```python
from build123d import *

# Parameters (mm, degrees)
EXTRUDE_1_DEPTH             = 25
EXTRUDE_3_DEPTH             = 25
CUT_EXTRUDE_1_DEPTH         = 53.179559149
CUT_EXTRUDE_1_DEPTH_BACK    = 53.179559149
SKETCH_4_W                  = 32
SKETCH_4_H                  = 14.912747354
FILLET_1_R                  = 10
FILLET_17_R                 = 2
CUT_EXTRUDE_5_DEPTH         = 60.625850278
CUT_EXTRUDE_5_DEPTH_BACK    = 60.625850278
CUT_EXTRUDE_6_DEPTH         = 60.600832153
CUT_EXTRUDE_6_DEPTH_BACK    = 60.600832153
SKETCH_9_W                  = 7
SKETCH_9_H                  = 3
SKETCH_10_W                 = 4.226496159
SKETCH_10_H                 = 9
EXTRUDE_4_DEPTH             = 10
SKETCH_12_W                 = 50
SKETCH_12_H                 = 3
EXTRUDE_6_DEPTH             = 10
EXTRUDE_6_DIRECTION_2_REACH = 62.659
SKETCH_14_R                 = 1
CUT_EXTRUDE_8_DEPTH         = 64.621818473
FILLET_50_R                 = 1.32
SKETCH_16_W                 = 32
SKETCH_16_H                 = 21.912747354
EXTRUDE_7_DEPTH             = 4.226496158
EXTRUDE_START               = 32
EXTRUDE_8_DEPTH             = 32
CHAMFER_1_SIZE              = 3


with BuildPart() as part:
    # 草图1 → 凸台-拉伸1 (new, symmetric)
    with BuildSketch(Plane.XY):
        with BuildLine():
            ThreePointArc((-33, 0), (-29.908156972, 13.946402637), (-21.21199112, 25.279466623))
            Line((-21.21199112, 25.279466623), (-16.985494961, 24.909696123))
            Line((-16.985494961, 24.909696123), (-19.283628291, 22.981333294))
            ThreePointArc((-19.283628291, 22.981333294), (-27.189233611, 12.678547852), (-30, 0))
            Line((-30, 0), (-33, 0))
        make_face()
    extrude(amount=EXTRUDE_1_DEPTH, both=True)

    # 草图1<7> → 凸台-拉伸3 (add, symmetric)
    with BuildSketch(Plane.XY):
        Polygon((-21.21199112, 25.279466623), (-21.21199112, 39.909696123), (-28.21199112, 39.909696123), (-28.21199112, 42.909696123), (-16.985494961, 42.909696123), (-16.985494961, 39.909696123), (-16.985494961, 24.909696123), align=None)
    extrude(amount=EXTRUDE_3_DEPTH, both=True)

    # 草图4 → 切除-拉伸1 (cut, two sides: drawn at the far end of the back side and taken through both)
    with BuildSketch(Plane(origin=(-16.985494961, 0, 0), x_dir=(0, 0, -1), z_dir=(1, 0, 0)).offset(-CUT_EXTRUDE_1_DEPTH_BACK)):
        with Locations((0, 35.453322446)):
            Rectangle(SKETCH_4_W, SKETCH_4_H)
    extrude(amount=CUT_EXTRUDE_1_DEPTH + CUT_EXTRUDE_1_DEPTH_BACK, mode=Mode.SUBTRACT)

    # 圆角1
    # the kernel refuses this fillet: 10 mm, written as the material it adds along each edge
    with BuildSketch(Plane(origin=(-21.21199112, 25.279466623, 25), x_dir=(-0.7281290100330119, -0.6854401102564294, 0), z_dir=(0, 0, -1))) as fillet_1_piece_1_section:
        with BuildLine():
            CenterArc((4.335441405, 9.983715921), FILLET_1_R, 223.270229162, 43.459541677)
            Line((-2.945848695, 3.129314818), (0, 0))
            ThreePointArc((0, 0), (1.882494294, 0.053737462), (3.764988589, 0))
        make_face()
    fillet_1_piece_1 = extrude(amount=50, mode=Mode.PRIVATE)
    fillet_1_piece_1 = split(fillet_1_piece_1, bisect_by=Plane(origin=(-21.85438977, 25.398045646, 16), z_dir=(0, 0, 1)), keep=Keep.TOP, mode=Mode.PRIVATE)
    fillet_1_piece_1 = split(fillet_1_piece_1, bisect_by=Plane(origin=(-21.85438977, 27.996948769, 20.5), z_dir=(0, -1, 0)), keep=Keep.TOP, mode=Mode.PRIVATE)
    add(fillet_1_piece_1)
    with BuildSketch(Plane(origin=(-21.21199112, 25.279466623, 25), x_dir=(-0.7281290100330119, -0.6854401102564294, 0), z_dir=(0, 0, -1))) as fillet_1_piece_2_section:
        with BuildLine():
            CenterArc((4.335441405, 9.983715921), FILLET_1_R, 223.270229162, 43.459541677)
            Line((-2.945848695, 3.129314818), (0, 0))
            ThreePointArc((0, 0), (1.882494294, 0.053737462), (3.764988589, 0))
        make_face()
    fillet_1_piece_2 = extrude(amount=50, mode=Mode.PRIVATE)
    fillet_1_piece_2 = split(fillet_1_piece_2, bisect_by=Plane(origin=(-21.135777092, 28.718730095, 16), z_dir=(0, 0, 1)), keep=Keep.TOP, mode=Mode.PRIVATE)
    fillet_1_piece_2 = split(fillet_1_piece_2, bisect_by=Plane(origin=(-21.135777092, 27.996948769, 20.5), z_dir=(0, 1, 0)), keep=Keep.TOP, mode=Mode.PRIVATE)
    add(fillet_1_piece_2)
    with BuildSketch(Plane(origin=(-21.21199112, 25.279466623, 25), x_dir=(-0.7281290100330119, -0.6854401102564294, 0), z_dir=(0, 0, -1))) as fillet_1_piece_3_section:
        with BuildLine():
            CenterArc((4.335441405, 9.983715921), FILLET_1_R, 223.270229162, 43.459541677)
            Line((-2.945848695, 3.129314818), (0, 0))
            ThreePointArc((0, 0), (1.882494294, 0.053737462), (3.764988589, 0))
        make_face()
    fillet_1_piece_3 = extrude(amount=50, mode=Mode.PRIVATE)
    fillet_1_piece_3 = split(fillet_1_piece_3, bisect_by=Plane(origin=(-21.85438977, 25.398045646, 16), z_dir=(0, 0, -1)), keep=Keep.TOP, mode=Mode.PRIVATE)
    fillet_1_piece_3 = split(fillet_1_piece_3, bisect_by=Plane(origin=(-21.85438977, 27.996948769, 0), z_dir=(0, -1, 0)), keep=Keep.TOP, mode=Mode.PRIVATE)
    fillet_1_piece_3 = split(fillet_1_piece_3, bisect_by=Plane(origin=(-21.85438977, 25.398045646, -16), z_dir=(0, 0, 1)), keep=Keep.TOP, mode=Mode.PRIVATE)
    add(fillet_1_piece_3)
    with BuildSketch(Plane(origin=(-21.21199112, 25.279466623, 25), x_dir=(-0.7281290100330119, -0.6854401102564294, 0), z_dir=(0, 0, -1))) as fillet_1_piece_4_section:
        with BuildLine():
            CenterArc((4.335441405, 9.983715921), FILLET_1_R, 223.270229162, 43.459541677)
            Line((-2.945848695, 3.129314818), (0, 0))
            ThreePointArc((0, 0), (1.882494294, 0.053737462), (3.764988589, 0))
        make_face()
    fillet_1_piece_4 = extrude(amount=50, mode=Mode.PRIVATE)
    fillet_1_piece_4 = split(fillet_1_piece_4, bisect_by=Plane(origin=(-21.85438977, 27.996948769, -20.5), z_dir=(0, -1, 0)), keep=Keep.TOP, mode=Mode.PRIVATE)
    fillet_1_piece_4 = split(fillet_1_piece_4, bisect_by=Plane(origin=(-21.85438977, 25.398045646, -16), z_dir=(0, 0, -1)), keep=Keep.TOP, mode=Mode.PRIVATE)
    add(fillet_1_piece_4)
    with BuildSketch(Plane(origin=(-21.21199112, 25.279466623, 25), x_dir=(-0.7281290100330119, -0.6854401102564294, 0), z_dir=(0, 0, -1))) as fillet_1_piece_5_section:
        with BuildLine():
            CenterArc((4.335441405, 9.983715921), FILLET_1_R, 223.270229162, 43.459541677)
            Line((-2.945848695, 3.129314818), (0, 0))
            ThreePointArc((0, 0), (1.882494294, 0.053737462), (3.764988589, 0))
        make_face()
    fillet_1_piece_5 = extrude(amount=50, mode=Mode.PRIVATE)
    fillet_1_piece_5 = split(fillet_1_piece_5, bisect_by=Plane(origin=(-21.135777092, 27.996948769, -20.5), z_dir=(0, 1, 0)), keep=Keep.TOP, mode=Mode.PRIVATE)
    fillet_1_piece_5 = split(fillet_1_piece_5, bisect_by=Plane(origin=(-21.135777092, 28.718730095, -16), z_dir=(0, 0, -1)), keep=Keep.TOP, mode=Mode.PRIVATE)
    add(fillet_1_piece_5)

    # 圆角17
    fillet_17_edges = [part.edges().sort_by_distance(p)[0] for p in [
        (-16.985494961, 24.909696123, 0),
    ]]
    fillet(fillet_17_edges, radius=FILLET_17_R)

    # 草图7 → 切除-拉伸5 (cut, two sides: drawn at the far end of the back side and taken through both)
    with BuildSketch(Plane.XY.offset(-CUT_EXTRUDE_5_DEPTH_BACK)):
        with BuildLine():
            Line((0, 0), (-33, 0))
            ThreePointArc((-33, 0), (-32.988691724, 0.863839294), (-32.954774647, 1.727086556))
            Line((-32.954774647, 1.727086556), (0, 0))
        make_face()
    extrude(amount=CUT_EXTRUDE_5_DEPTH + CUT_EXTRUDE_5_DEPTH_BACK, mode=Mode.SUBTRACT)

    # 草图9 → 切除-拉伸6 (cut, two sides: drawn at the far end of the back side and taken through both)
    with BuildSketch(Plane.XY.offset(-CUT_EXTRUDE_6_DEPTH_BACK)):
        with Locations((-24.71199112, 41.409696123)):
            Rectangle(SKETCH_9_W, SKETCH_9_H)
    extrude(amount=CUT_EXTRUDE_6_DEPTH + CUT_EXTRUDE_6_DEPTH_BACK, mode=Mode.SUBTRACT)

    # 草图10 → 凸台-拉伸4 (add)
    with BuildSketch(Plane(origin=(0, 42.909696123, 0), x_dir=(1, 0, 0), z_dir=(0, 1, 0))):
        with Locations((-19.098743041, 20.5)):
            Rectangle(SKETCH_10_W, SKETCH_10_H)
        with Locations((-19.098743041, -20.5)):
            Rectangle(SKETCH_10_W, SKETCH_10_H)
    extrude(amount=EXTRUDE_4_DEPTH)

    # 草图12 → 凸台-拉伸6 (add)
    with BuildSketch(Plane(origin=(-16.985494961, 0, 0), x_dir=(0, 0, -1), z_dir=(1, 0, 0))):
        with Locations((0, 51.409696123)):
            Rectangle(SKETCH_12_W, SKETCH_12_H)
    extrude(amount=EXTRUDE_6_DEPTH)

    # 凸台-拉伸6 direction 2: up to this face of the body (flat: up to its plane)
    extrude_6_direction_2_end = Plane(part.part.faces().sort_by_distance((-21.21199112, 41.24345525, 20.5))[0])
    # 草图12 → 凸台-拉伸6 direction 2 (add, up to the picked face)
    with BuildSketch(Plane(origin=(-16.985494961, 0, 0), x_dir=(0, 0, -1), z_dir=(1, 0, 0)), mode=Mode.PRIVATE) as extrude_6_direction_2_sk1:
        with Locations((0, 51.409696123)):
            Rectangle(SKETCH_12_W, SKETCH_12_H)
    extrude_6_direction_2_tool1 = split(extrude(extrude_6_direction_2_sk1.sketch, amount=-EXTRUDE_6_DIRECTION_2_REACH, mode=Mode.PRIVATE), bisect_by=extrude_6_direction_2_end, keep=Keep.BOTH, mode=Mode.PRIVATE)
    add(extrude_6_direction_2_tool1.solids().sort_by(Axis((-16.985495, 51.409696, 0), (-1, 0, 0)))[0])

    # 草图14 → 切除-拉伸8 (cut, through all)
    with BuildSketch(Plane(origin=(0, 49.909696123, 0), x_dir=(-1, 0, 0), z_dir=(0, -1, 0))):
        with Locations(Location((10.985494961, 19, 0), (0, 0, 180))):
            Circle(SKETCH_14_R)
        with Locations((10.985494961, -19)):
            Circle(SKETCH_14_R)
    extrude(amount=-CUT_EXTRUDE_8_DEPTH, mode=Mode.SUBTRACT)

    # 圆角50
    fillet_50_edges = [part.edges().sort_by_distance(p)[0] for p in [
        (-21.21199112, 41.24345525, -25),
        (-21.21199112, 41.24345525, 25),
        (-21.922587859, 25.874919539, -25),
        (-21.922587859, 25.874919539, 25),
        (-30.324707269, 13.015841465, -25),
        (-30.324707269, 13.015841465, 25),
        (-29.958886043, 1.570078687, 0),
        (-32.954774647, 1.727086556, 0),
    ]]
    fillet(fillet_50_edges, radius=FILLET_50_R)

    # 草图16 → 凸台-拉伸7 (add)
    with BuildSketch(Plane(origin=(-16.985494961, 0, 0), x_dir=(0, 0, -1), z_dir=(1, 0, 0))):
        with Locations((0, 38.953322446)):
            Rectangle(SKETCH_16_W, SKETCH_16_H)
    extrude(amount=-EXTRUDE_7_DEPTH)

    # 草图17 → 凸台-拉伸8 (add)
    with BuildSketch(Plane.XY.offset(-16).offset(EXTRUDE_START)):
        with BuildLine():
            Line((-21.337642503, 27.996948769), (-21.21199112, 27.996948769))
            Line((-21.21199112, 27.996948769), (-21.21199112, 29.577214378))
            ThreePointArc((-21.21199112, 29.577214378), (-21.243453459, 28.784587785), (-21.337642503, 27.996948769))
        make_face()
    extrude(amount=-EXTRUDE_8_DEPTH)

    # 倒角1
    chamfer_1_edges = [part.edges().sort_by_distance(p)[0] for p in [
        (-16.985494961, 49.909696123, 0),
    ]]
    chamfer(chamfer_1_edges, length=CHAMFER_1_SIZE)


solid = part.part
```
Design review of the part built by this model. Coordinates are the model's own, in mm. A direction names the side the tool comes from. Give positions to 0.01 mm unless a question says otherwise; leave off trailing zeros. Write each loop counter-clockwise with the first axis right and the second up, starting at its lowest first coordinate (ties: lowest second). Pieces come first, ordered by that corner, then holes. Notation, with made-up numbers: (26.25, 33) - (43.25, 33) arc R16 cw to (43.25, 47) - close; hole circle Ø4 at (60, 33.5). An arc over 180 degrees is marked (long way). Return JSON: item names as keys, results as strings. Group by question number.
(1) We need section B-B, the plane z = 6.5. Give the boundary of the cut face in (x, y), then the cut area to 3 significant figures.
(2) Machinability: for faces 1 (the flat face through (-16.985, 37, 0)), 2 (the flat face through (-21.212, 41, 0)), 3 (the flat face through (-19, 35, -25)), which of the approach directions +Z, -Z, +X, -X, +Y, -Y give a long, thin tool a straight path to every point of the face, cutting with its end or side? Answer none if there is none.
(3) To check wall thickness, follow probe 1 along X at (y, z) = (51, 19); probe 2 along Y at (x, z) = (-11.5, -13); probe 3 along X at (y, z) = (40, 14.5). State the ranges of each line that lie inside material, in increasing order.
(4) We need section C-C, the plane x = -13. Give the boundary of the cut face in (y, z).
(5) Mouldability with a two-part tool opening along X and no side actions: class faces 4 (the flat face through (-18.481, 23.655, 0.35)), 5 (the flat face through (-19, 35, 25)), 6 (the cylindrical face through (-10.192, 51.389, 19.608)) as +X half, -X half, draft (parallel to the pull), parting line (faces both ways), or undercut.
(6) We need section D-D, the plane x = -15.75. Give the boundary of the cut face in (y, z), then the cut area to 3 significant figures.
(7) We need section A-A, the plane z = 19. Give the boundary of the cut face in (x, y).
(8) Insertion check: pin 1 (2 mm diameter, centred on y = 37.5, z = 14, fed in from +X); pin 2 (4 mm diameter, centred on y = 39, z = 2, fed in from -X); pin 3 (2 mm diameter, centred on x = -11, z = -8.5, fed in from -Y); pin 4 (2 mm diameter, centred on x = -24, y = 36, fed in from -Z). Each pin has a flat end and moves straight along its axis. Give the tip position at first contact, or say it passes through.
Reported:
{
 "1": {"outline": "(-32.85, 3.1) arc R1.32 ccw to (-31.61, 1.66) - (-31.25, 1.64) arc R1.32 ccw to (-29.87, 2.83) arc R30 cw to (-19.28, 22.98) - (-17.7, 24.31) arc R2 ccw to (-16.99, 25.84) - (-16.99, 46.91) - (-13.99, 49.91) - (-6.99, 49.91) - (-6.99, 52.91) - (-21.21, 52.91) - (-21.21, 29.58) arc R10 cw to (-23.95, 22.7) arc R33 ccw to start", "area": "235 mm2"},
 "2": {"face 1": "+Z, -Z, +X, -Y", "face 2": "+Z, -Z, -X, +Y", "face 3": "-Z, +X, -X, +Y, -Y"},
 "3": {"probe 1": "x = -21.21 to -11.99, -9.99 to -6.99", "probe 2": "y = 49.91 to 52.91", "probe 3": "x = -21.21 to -16.99"},
 "4": {"outline": "(49.91, -25) - (52.91, -25) - (52.91, 25) - (49.91, 25) - close"},
 "5": {"face 4": "+X half", "face 5": "draft", "face 6": "undercut"},
 "6": {"outline": "(48.15, -25) - (52.91, -25) - (52.91, 25) - (48.15, 25) - close", "area": "238 mm2"},
 "7": {"outline": "(-32.85, 3.1) arc R1.32 ccw to (-31.61, 1.66) - (-31.25, 1.64) arc R1.32 ccw to (-29.87, 2.83) arc R30 cw to (-19.28, 22.98) - (-17.7, 24.31) arc R2 ccw to (-16.99, 25.84) - (-16.99, 46.91) - (-13.99, 49.91) - (-11.99, 49.91) - (-11.99, 52.91) - (-21.21, 52.91) - (-21.21, 29.58) arc R10 cw to (-23.95, 22.7) arc R33 ccw to start; (-9.99, 49.91) - (-6.99, 49.91) - (-6.99, 52.91) - (-9.99, 52.91) - close"},
 "8": {"pin 1": "stops at x = -16.99", "pin 2": "stops at x = -21.21", "pin 3": "stops at y = 49.91", "pin 4": "passes through"}
}
